from build123d import *

# Parameters (mm, degrees)
SKETCH1_W                   = 70
SKETCH1_H                   = 44
MIAN_BOSS_EXTRUDE_DEPTH     = 30
SKETCH2_W                   = 60
SKETCH2_H                   = 36
MAIN_CUT_DEPTH              = 15
SKETCH4_W                   = 45
SKETCH4_H                   = 35
BATTERY_CUT_DEPTH           = 9
SKETCH5_R                   = 6.375
ELCTRODE_CUT_DEPTH          = 18
SKETCH6_W                   = 10
SKETCH6_H                   = 24.5
USB_C_CUT_DEPTH             = 7
SKETCH7_R                   = 3.625
BUTTON_CUT_DEPTH            = 7
SKETCH8_W                   = 9
SKETCH8_H                   = 4
SWITCH_CUT_DEPTH            = 7
OUTSIDE_FILLET_R            = 2.5
SKETCH10_OUTSIDE_W          = 89.59
SKETCH10_OUTSIDE_H          = 63.59
SKETCH10_OUTSIDE_W_2        = 66
SKETCH10_OUTSIDE_H_2        = 40
OUTER_LID_EXTRUDE_DEPTH     = 4
LID_SNAP_EXTRUDE_DEPTH      = 1
LID_SNAP_EXTRUDE_DEPTH_BACK = 41
SKETCH11_W                  = 5
SKETCH11_H                  = 2
SKETCH13_W                  = 11
SKETCH13_H                  = 36
INNER_LID_EXTRUDE_DEPTH     = 3
SKETCH14_W                  = 14
SKETCH14_H                  = 26.5
SKETCH14_W_2                = 10
SKETCH14_H_2                = 24.5
USB_COVER_EXTRUDE_DEPTH     = 3
SKETCH15_W                  = 4
SKETCH15_H                  = 9
BUTTON_SIDE_CUT_DEPTH       = 1
CHAMFER1_SIZE               = 10
LID_SNAP_FILLET_R           = 0.5


with BuildPart() as part:
    # Sketch1 → Mian Boss Extrude (new body)
    with BuildSketch(Plane.XY):
        with Locations((35, 22)):
            Rectangle(SKETCH1_W, SKETCH1_H)
    extrude(amount=MIAN_BOSS_EXTRUDE_DEPTH)

    # Sketch2 → Main cut (cut)
    with BuildSketch(Plane.XY.offset(30)):
        with Locations((34, 22)):
            Rectangle(SKETCH2_W, SKETCH2_H)
    extrude(amount=-MAIN_CUT_DEPTH, mode=Mode.SUBTRACT)

    # Sketch4 → Battery Cut (cut)
    with BuildSketch(Plane.XY.offset(15)):
        with Locations((34, 21.5)):
            Rectangle(SKETCH4_W, SKETCH4_H)
    extrude(amount=-BATTERY_CUT_DEPTH, mode=Mode.SUBTRACT)

    # Sketch5 → Elctrode Cut (cut)
    with BuildSketch(Plane(origin=(0, 0, 0), x_dir=(-1, 0, 0), z_dir=(0, 0, -1))):
        with Locations((-59.25, 23)):
            Circle(SKETCH5_R)
        with Locations((-12.75, 23)):
            Circle(SKETCH5_R)
    extrude(amount=-ELCTRODE_CUT_DEPTH, mode=Mode.SUBTRACT)

    # Sketch6 → USB-c Cut (cut)
    with BuildSketch(Plane(origin=(70, 0, 0), x_dir=(0, 0, -1), z_dir=(1, 0, 0))):
        with Locations((-20, 27.75)):
            Rectangle(SKETCH6_W, SKETCH6_H)
    extrude(amount=-USB_C_CUT_DEPTH, mode=Mode.SUBTRACT)

    # Sketch7 → Button Cut (cut)
    with BuildSketch(Plane.ZY):
        with Locations((21.5, 8)):
            Circle(SKETCH7_R)
    extrude(amount=-BUTTON_CUT_DEPTH, mode=Mode.SUBTRACT)

    # Sketch8 → Switch Cut (cut)
    with BuildSketch(Plane.XZ):
        with Locations((38.5, 17)):
            Rectangle(SKETCH8_W, SKETCH8_H)
    extrude(amount=-SWITCH_CUT_DEPTH, mode=Mode.SUBTRACT)

    # Outside Fillet
    outside_fillet_edges = [part.edges().sort_by_distance(p)[0] for p in [
        (0, 44, 15),
        (70, 44, 15),
        (70, 0, 15),
        (0, 0, 15),
    ]]
    fillet(outside_fillet_edges, radius=OUTSIDE_FILLET_R)

    # Sketch10 outside → Outer lid Extrude (cut)
    with BuildSketch(Plane.XY.offset(30)):
        with Locations((35, 22)):
            Rectangle(SKETCH10_OUTSIDE_W, SKETCH10_OUTSIDE_H)
        with Locations((35, 22)):
            Rectangle(SKETCH10_OUTSIDE_W_2, SKETCH10_OUTSIDE_H_2, mode=Mode.SUBTRACT)
    extrude(amount=-OUTER_LID_EXTRUDE_DEPTH, mode=Mode.SUBTRACT)

    # Sketch11 → Lid Snap-Extrude (add, two sides: drawn at the far end of the back side and taken through both)
    with BuildSketch(Plane.XZ.offset(-2).offset(-LID_SNAP_EXTRUDE_DEPTH_BACK)):
        with Locations((31, 28)):
            Rectangle(SKETCH11_W, SKETCH11_H)
        with Locations((37, 28)):
            Rectangle(SKETCH11_W, SKETCH11_H)
    extrude(amount=LID_SNAP_EXTRUDE_DEPTH + LID_SNAP_EXTRUDE_DEPTH_BACK)

    # Sketch13 → Inner Lid-Extrude (cut)
    with BuildSketch(Plane.XY.offset(29)):
        with Locations((34, 22)):
            Rectangle(SKETCH13_W, SKETCH13_H)
    extrude(amount=-INNER_LID_EXTRUDE_DEPTH, mode=Mode.SUBTRACT)

    # Sketch14 → USB Cover-Extrude (add)
    with BuildSketch(Plane(origin=(70, 0, 0), x_dir=(0, 0, -1), z_dir=(1, 0, 0))):
        with Locations((-19, 27.75)):
            Rectangle(SKETCH14_W, SKETCH14_H)
        with Locations((-20, 27.75)):
            Rectangle(SKETCH14_W_2, SKETCH14_H_2, mode=Mode.SUBTRACT)
    extrude(amount=USB_COVER_EXTRUDE_DEPTH)

    # Sketch15 → Button side cut (cut)
    with BuildSketch(Plane(origin=(0, 4, 0), x_dir=(1, 0, 0), z_dir=(0, 1, 0))):
        with Locations((6, -21.5)):
            Rectangle(SKETCH15_W, SKETCH15_H)
    extrude(amount=-BUTTON_SIDE_CUT_DEPTH, mode=Mode.SUBTRACT)

    # Chamfer1
    # the kernel refuses this chamfer: 10 mm, written as the material it takes off along each edge
    with BuildSketch(Plane(origin=(8, 4, 17), x_dir=(0.9996219169112968, 0.027495876610586403, 0), z_dir=(0, 0, 1))) as chamfer1_piece_1_section:
        Polygon((CHAMFER1_SIZE * 0.999621916911, -CHAMFER1_SIZE * 0.0274958766106), (-CHAMFER1_SIZE * 0.0274958766106, -CHAMFER1_SIZE * 0.999621916911), (0, 0), align=None)
    chamfer1_piece_1 = extrude(amount=9, mode=Mode.PRIVATE)
    chamfer1_piece_1 = split(chamfer1_piece_1, bisect_by=Plane(origin=(14.506944444, 3, 21.5), z_dir=(0, 1, 0)), keep=Keep.TOP, mode=Mode.PRIVATE)
    add(chamfer1_piece_1, mode=Mode.SUBTRACT)

    # Lid Snap Fillet
    lid_snap_fillet_edges = [part.edges().sort_by_distance(p)[0] for p in [
        (28.5, 43, 28),
        (31, 43, 29),
        (33.5, 43, 28),
        (31, 43, 27),
        (28.5, 1, 28),
        (31, 1, 27),
        (33.5, 1, 28),
        (31, 1, 29),
        (37, 43, 29),
        (39.5, 43, 28),
        (37, 43, 27),
        (34.5, 43, 28),
        (37, 1, 29),
        (34.5, 1, 28),
        (37, 1, 27),
        (39.5, 1, 28),
    ]]
    fillet(lid_snap_fillet_edges, radius=LID_SNAP_FILLET_R)


solid = part.part
Could you check a few things on this model? Use its own coordinates, in mm. A direction names the side the tool comes from. Give positions to 0.01 mm unless a question says otherwise; leave off trailing zeros. Write each loop counter-clockwise with the first axis right and the second up, starting at its lowest first coordinate (ties: lowest second). Pieces come first, ordered by that corner, then holes. Notation, with made-up numbers: (87, 0.5) -> (126, 0.5) arc R35 cw to (126, 37.5) -> close; hole circle Ø5 at (-18.75, 30). An arc over 180 degrees is marked (long way). Answer as CSV lines item,"result". Start each with the question number.
(1) If we section it at C-C, the plane y = 35: Write out the boundary of the cut face in (x, z).
(2) If we mould it in two halves opening along Y, with no side actions, what happens to faces 5 (the face through (68, 22, 28)), 6 (the face through (4, 21, 23)), 7 (the face through (69.248, 43.287, 13.182))? For each: +Y half, -Y half, draft (parallel to the pull), parting line (faces both ways), or undercut.
(3) If we section it at A-A, the plane y = 23: Write out the boundary of the cut face in (x, z) (3 decimals).
(4) If we section it at D-D, the plane x = 12.75: Write out the boundary of the cut face in (y, z) (3 decimals), and give its area (4 significant figures).
(5) Which directions (+Z, -Z, +X, -X, +Y, -Y) give clear straight access to the entire face, cutting with the end or side of a thin tool? Please do faces 1 (the face through (40.9, 39.2, 15)), 2 (the face through (71, 14.5, 19)), 3 (the face through (64, 18, 26)), 4 (the face through (38, 2, 15)).
(6) If we section it at B-B, the plane z = 21.5: Write out the boundary of the cut face in (x, y) (3 decimals), and give its area (3 significant figures).
(7) Please list where these lines run through material, in increasing order: line 1 (X direction, y = 14, z = 7.75); line 2 (X direction, y = 23, z = 11.75) (3 decimals); line 3 (Y direction, x = 19, z = 18.5).
(8) I'm going to push flat-ended pins straight in: pin 1 Ø1 at (y, z) = (23.5, 20.5) entering from +X; pin 2 Ø6 at (x, y) = (23.5, 24) entering from +Z; pin 3 Ø3.5 at (x, z) = (72, 17) entering from +Y. Where does each tip first touch, or does it pass through?
Answer list:
1,outline,"(0, 0) -> (70, 0) -> (70, 12) -> (73, 12) -> (73, 15) -> (56.5, 15) -> (56.5, 6) -> (11.5, 6) -> (11.5, 15) -> (4, 15) -> (4, 30) -> (2, 30) -> (2, 26) -> (0, 26) -> close; (64, 25) -> (73, 25) -> (73, 26) -> (68, 26) -> (68, 30) -> (64, 30) -> close"
2,face 5,"draft"
2,face 6,"undercut"
2,face 7,"+Y half"
3,outline,"(0, 0) -> (6.375, 0) -> (6.375, 15) -> (4, 15) -> (4, 30) -> (2, 30) -> (2, 26) -> (0, 26) -> close; (19.125, 0) -> (52.875, 0) -> (52.875, 6) -> (19.125, 6) -> close; (64, 25) -> (73, 25) -> (73, 26) -> (68, 26) -> (68, 30) -> (64, 30) -> close; (65.625, 0) -> (70, 0) -> (70, 12) -> (73, 12) -> (73, 15) -> (65.625, 15) -> close"
4,outline,"(0, 0) -> (16.625, 0) -> (16.625, 6) -> (4, 6) -> (4, 17) -> (3, 17) -> (3, 26) -> (4, 26) -> (4, 30) -> (2, 30) -> (2, 26) -> (0, 26) -> close; (29.375, 0) -> (44, 0) -> (44, 26) -> (42, 26) -> (42, 30) -> (40, 30) -> (40, 15) -> (39, 15) -> (39, 6) -> (29.375, 6) -> close"
4,area,"363.5 mm^2"
5,face 1,"none"
5,face 2,"+Z, -Z, +X, -Y"
5,face 3,"+Z"
5,face 4,"-Y"
6,outline,"(0, 2.5) arc R2.5 ccw to (2.5, 0) -> (67.5, 0) arc R2.5 ccw to (70, 2.5) -> (70, 14.5) -> (73, 14.5) -> (73, 15.5) -> (64, 15.5) -> (64, 4) -> (18, 4) -> (17, 3) -> (4, 3) -> (4, 4.375) -> (0, 4.375) -> close; (0, 11.625) -> (4, 11.625) -> (4, 40) -> (73, 40) -> (73, 41) -> (70, 41) -> (70, 41.5) arc R2.5 ccw to (67.5, 44) -> (2.5, 44) arc R2.5 ccw to (0, 41.5) -> close"
6,area,"731 mm^2"
7,line 1,"0 to 11.5, 56.5 to 70"
7,line 2,"0 to 6.375, 65.625 to 70"
7,line 3,"0 to 4, 40 to 44"
8,pin 1,"x = 4"
8,pin 2,"z = 6"
8,pin 3,"y = 41"
